from build123d import *

# Parameters (mm, degrees)
PROFILEBOSS_EXTRUDE1_DEPTH           = 80
SKETCH2_R                            = 2.3
LEDSTRIPMOUNTHOLESCUT_EXTRUDE1_DEPTH = 4.5
SKETCH4_W                            = 28
SKETCH4_H                            = 11.5
POWERCONNECTORCUT_EXTRUDE4_DEPTH     = 6.5
SKETCH3_R                            = 2.3
MOUNTINGHOLESCUT_EXTRUDE3_DEPTH      = 4.5
SKETCH5_W                            = 80
SKETCH5_H                            = 2
XAXISCABLECUT_EXTRUDE1_DEPTH         = 4.25


with BuildPart() as part:
    # Sketch1 → ProfileBoss-Extrude1 (new body)
    with BuildSketch(Plane(origin=(0, 0, 0), x_dir=(0, 0, -1), z_dir=(1, 0, 0))):
        with BuildLine():
            Line((0, 0), (5.499461553, 0))
            ThreePointArc((5.499461553, 0), (6.914055855, 0.585944145), (7.5, 2.000538447))
            Line((7.5, 2.000538447), (7.5, 3.5))
            Line((7.5, 3.5), (17.922539551, 8.36011001))
            Line((17.922539551, 8.36011001), (19.190394336, 5.641186649))
            ThreePointArc((19.190394336, 5.641186649), (20.700753359, 6.16912635), (21.340729536, 7.635528477))
            Line((21.340729536, 7.635528477), (21.340729536, 13.36011001))
            ThreePointArc((21.340729536, 13.36011001), (20.754943098, 14.774323572), (19.340729536, 15.36011001))
            Line((19.340729536, 15.36011001), (0, 15.36011001))
            Line((0, 15.36011001), (0, 0))
        make_face()
    extrude(amount=PROFILEBOSS_EXTRUDE1_DEPTH)

    # Sketch2 → LedStripMountHolesCut-Extrude1 (cut)
    with BuildSketch(Plane(origin=(0, 0.002211655, 0.001031312), x_dir=(1, 0, 0), z_dir=(0, -0.906307787036651, -0.4226182617406973))):
        with Locations(Location((43.85, -14.026472319, 0), (0, 0, 270))):
            Circle(SKETCH2_R)
    extrude(amount=-LEDSTRIPMOUNTHOLESCUT_EXTRUDE1_DEPTH, mode=Mode.SUBTRACT)

    # Sketch4 → PowerConnectorCut-Extrude4 (cut)
    with BuildSketch(Plane(origin=(0, 0.002211655, 0.001031312), x_dir=(1, 0, 0), z_dir=(0, -0.906307787036651, -0.4226182617406973))):
        with Locations((66, -14.026472319)):
            Rectangle(SKETCH4_W, SKETCH4_H)
    extrude(amount=-POWERCONNECTORCUT_EXTRUDE4_DEPTH, mode=Mode.SUBTRACT)

    # Sketch3 → MountingHolesCut-Extrude3 (cut)
    with BuildSketch(Plane.XY):
        with Locations((30, 10.86011001)):
            Circle(SKETCH3_R)
    extrude(amount=-MOUNTINGHOLESCUT_EXTRUDE3_DEPTH, mode=Mode.SUBTRACT)

    # Sketch5 → XAxisCableCut-Extrude1 (cut)
    with BuildSketch(Plane.XY):
        with Locations((40, 3.5)):
            Rectangle(SKETCH5_W, SKETCH5_H)
    extrude(amount=-XAXISCABLECUT_EXTRUDE1_DEPTH, mode=Mode.SUBTRACT)


solid = part.part
Verification items for the finished model (mm, model axes). A direction names the side the tool comes from. Coordinates: 2 decimals unless noted, no trailing zeros. Order: outer loops, then holes, each group sorted by start corner. A loop starts at its lowest first (then second) coordinate and runs counter-clockwise, first axis right, second up. Notation, with made-up numbers: M -37.75,73 L -12.75,73 A30 cw -12.75,95 Z; hole C 0,12.25 d9. An arc over 180 degrees is marked long. One line per item, written item: value. Start each with the question number.
Item 1: Gauge pin test, flat ends, axial feed: pin 1 (6 mm diameter, centred on x = 69.5, y = 3, fed in from -Z); pin 2 (1.4 mm diameter, centred on x = 30.5, y = 12, fed in from +Z); pin 3 (1.2 mm diameter, centred on x = 51, y = 3, fed in from -Z). Record the tip position at first contact, or that the pin passes through.
Item 2: Sectioned sample at C-C (z = -6.25). Enter the section's corners in (x, y), then the cut area to 3 significant figures.
Item 3: Sectioned sample at A-A (z = -1.5). Enter the section's corners in (x, y), then the cut area to 3 significant figures.
Item 4: Scan lines: probe 1 along Y at (x, z) = (30, -1.3); probe 2 along X at (y, z) = (10.75, -3.5); probe 3 along X at (y, z) = (8, -5.75). Record each from-to range of solid material in increasing order.
Item 5: Sectioned sample at B-B (x = 62). Enter the section's corners in (y, z).
Item 6: Mould release check, pull along Y, two halves, no side actions. Record for faces 1 (the cylindrical face through (39.44, 0.57, -6.9)), 2 (the flat face through (39, 10, 0)), 3 (the flat face through (65.804, 11.787, -9.891)): released by +Y, released by -Y, zero draft, split by the parting line, or undercut.
Item 7: Access from +Z, -Z, +X, -X, +Y, -Y to the whole of each face (thin tool, end or side, straight path). Record for faces 4 (the flat face through (39, 4, -4.25)), 5 (the flat face through (30, 11, -4.5)), 6 (the flat face through (65.804, 6.404, -6.146)).
Item 8: Sectioned sample at D-D (x = 10). Enter the section's corners in (y, z).
Conclusion:
1. pin 1: stops at z = -20.49
1. pin 2: stops at z = -4.5
1. pin 3: stops at z = -7.71
2. outline: M 0,0.15 L 80,0.15 L 80,6.18 L 52,6.18 L 52,10.09 L 80,10.09 L 80,15.36 L 0,15.36 Z
2. area: 1,110 mm^2
3. outline: M 0,0 L 80,0 L 80,2.5 L 0,2.5 Z; M 0,4.5 L 80,4.5 L 80,15.36 L 0,15.36 Z; hole C 30,10.86 d4.6
3. area: 1,050 mm^2
4. probe 1: y = 0 to 2.5, 4.5 to 8.56, 13.16 to 15.36
4. probe 2: x = 0 to 27.7, 32.3 to 80
4. probe 3: x = 0 to 52
5. outline: M 0,-5.5 A2 ccw 2,-7.5 L 3.5,-7.5 L 9.39,-4.75 L 14.25,-15.18 L 5.64,-19.19 A2 ccw 7.64,-21.34 L 13.36,-21.34 A2 ccw 15.36,-19.34 L 15.36,0 L 4.5,0 L 4.5,-4.25 L 2.5,-4.25 L 2.5,0 L 0,0 Z
6. face 1: released by -Y
6. face 2: zero draft
6. face 3: undercut
7. face 4: +Z, +X, -X
7. face 5: +Z
7. face 6: +X
8. outline: M 0,-5.5 A2 ccw 2,-7.5 L 3.5,-7.5 L 8.36,-17.92 L 5.64,-19.19 A2 ccw 7.64,-21.34 L 13.36,-21.34 A2 ccw 15.36,-19.34 L 15.36,0 L 4.5,0 L 4.5,-4.25 L 2.5,-4.25 L 2.5,0 L 0,0 Z
